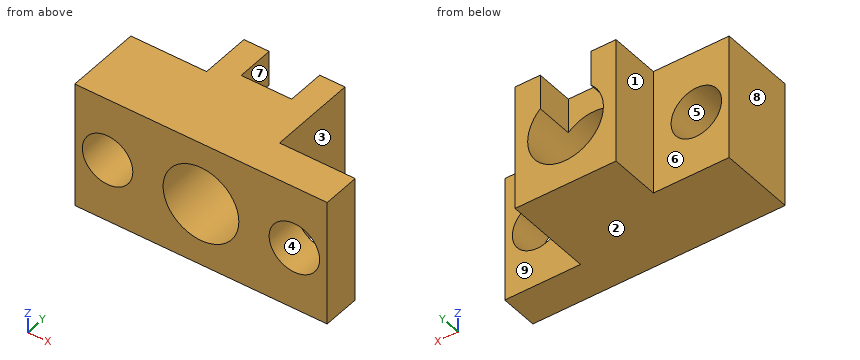
Autodesk Inventor part; units mm, degrees
ref_plane "YZ Plane" through (0, 0, 0) normal (1, 0, 0) x (0, 1, 0)
ref_plane "XZ Plane" through (0, 0, 0) normal (0, 1, 0) x (-1, 0, 0)
ref_plane "XY Plane" through (0, 0, 0) normal (0, 0, 1) x (1, 0, 0)
sketch "Sketch1" plane through (0, 0, 0) normal (0, 0, 1) x (1, 0, 0)
  line L0 (0, 0) -> (100, 0)
  line L1 (100, 0) -> (100, 15)
  line L2 (100, 15) -> (70, 15)
  line L3 (70, 15) -> (70, 50)
  line L4 (70, 50) -> (30, 50)
  line L5 (30, 50) -> (30, 30)
  line L6 (30, 30) -> (0, 30)
  line L7 (0, 30) -> (0, 0)
  dimension "d0" = 100
  dimension "d1" = 15
  dimension "d2" = 30
  dimension "d3" = 35
extrude "Extrusion1" add sketch "Sketch1" along normal blind 50
sketch "Sketch2" plane through (0, 0, 0) normal (0, -1, 0) x (1, 0, 0)
  circle A0 centre (13, 25) radius 10
  circle A1 centre (87, 25) radius 10
  circle A2 centre (50, 25) radius 15
  point P0 (0, 0)
extrude "Extrusion2" cut sketch "Sketch2" against normal blind 50
sketch "Sketch3" plane through (0, 0, 50) normal (0, 0, 1) x (1, 0, 0)
  line L0 (70, 50) -> (30, 50)
  line L1 (40, 50) -> (40, 35)
  line L2 (40, 35) -> (60, 35)
  line L3 (60, 35) -> (60, 50)
  line L4 (40, 50) -> (60, 50)
  line L5 (35, 50) -> (65, 50)
  point P0 (0, 0)
extrude "Extrusion3" cut sketch "Sketch3" against normal blind 15
properties part number "P3-10"
Geometry: final body of the model. Coordinates: model frame, mm. Face numbers are marked on the shaded views. A direction names the side the tool comes from. Coordinates: 2 decimals unless noted, no trailing zeros. Write each loop counter-clockwise with the first axis right and the second up, starting at its lowest first coordinate (ties: lowest second). Pieces come first, ordered by that corner, then holes. Notation, with made-up numbers: M 11.25,18.5 L 63.25,18.5 A14 cw 63.25,28.5 Z; hole C -23,-12 d2. An arc over 180 degrees is marked long. Use CSV: the item, a comma, the result in double quotes. Start each with the question number.
1. Mould query, pull axis X, two halves, no side actions, for the marked faces 1, 2, 3 and 4. Classes: pulls with the +X half, pulls with the -X half, needs draft (parallel to the pull), parting line crosses it, or undercut.
2. Cut plane B-B on x = 50. Return the cut outline in (y, z), plus the area to 3 significant figures.
3. Cut plane D-D on z = 25. Return the cut outline in (x, y), plus the area to 3 significant figures.
4. Reachability of the marked faces 5, 6, 7, 8 and 9 from +Z, -Z, +X, -X, +Y, -Y: full face, straight path, thin tool, end or side. Return the list, or none.
5. Ray query, probe 1 along Z at (x, y) = (87, 3.5); probe 2 along X at (y, z) = (39, 45.5); probe 3 along Y at (x, z) = (29, 23). Return the intervals inside material, ascending.
6. Cut plane A-A on z = 13. Return the cut outline in (x, y), plus the area to 3 significant figures.
7. Cut plane C-C on y = 3. Return the cut outline in (x, z).
8. First-contact query: P1, Ø11, axis at y = 44.5, z = 46.5, coming from the +X side; P2, Ø11, axis at x = 46, z = 45.5, coming from the +Y side; P3, Ø6, axis at y = 35.5, z = 26, coming from the -X side. Flat tips, straight axial feed; report the tip coordinate or a pass-through.
Entries:
1,face 1,"pulls with the -X half"
1,face 2,"needs draft"
1,face 3,"pulls with the +X half"
1,face 4,"undercut"
2,outline,"M 0,0 L 50,0 L 50,10 L 0,10 Z; M 0,40 L 35,40 L 35,50 L 0,50 Z"
2,area,"850 mm²"
3,outline,"M 0,0 L 3,0 L 3,30 L 0,30 Z; M 23,0 L 35,0 L 35,50 L 30,50 L 30,30 L 23,30 Z; M 65,0 L 77,0 L 77,15 L 70,15 L 70,50 L 65,50 Z; M 97,0 L 100,0 L 100,15 L 97,15 Z"
3,area,"950 mm²"
4,face 5,"+Y, -Y"
4,face 6,"+Z, -Z, -X, +Y"
4,face 7,"+Z, +Y"
4,face 8,"+Z, -Z, -X, +Y, -Y"
4,face 9,"+Z, -Z, +X, +Y"
5,probe 1,"0 to 15, 35 to 50"
5,probe 2,"30 to 40, 60 to 70"
5,probe 3,"0 to 30"
6,outline,"M 0,0 L 41,0 L 41,50 L 30,50 L 30,30 L 0,30 Z; M 59,0 L 100,0 L 100,15 L 70,15 L 70,50 L 59,50 Z"
6,area,"2,450 mm²"
7,outline,"M 0,0 L 100,0 L 100,50 L 0,50 Z; hole C 13,25 d20; hole C 50,25 d30; hole C 87,25 d20"
8,P1,"x = 70"
8,P2,"y = 35"
8,P3,"x = 30"
